Check sheet for the modelled part. Datum: model origin and axes. Units: mm. A direction names the side the tool comes from. Coordinates: 2 decimals unless noted, no trailing zeros. Write each loop counter-clockwise with the first axis right and the second up, starting at its lowest first coordinate (ties: lowest second). Pieces come first, ordered by that corner, then holes. Notation, with made-up numbers: M 62,51 L 66,51 A15 ccw 66,55 Z; hole C -18.5,-26 d11. An arc over 180 degrees is marked long. Answer as CSV lines item,"result". Start each with the question number.
1) Go/stop test with flat-tipped pins: pin 1 Ø10 at (x, z) = (-9.5, 1.5) entering from -Y; pin 2 Ø3 at (x, z) = (1.5, -3) entering from +Y; pin 3 Ø1.5 at (x, y) = (-16.5, -7.5) entering from -Z. Record where each tip stops, or that it passes through.
2) Access from +Z, -Z, +X, -X, +Y, -Y to the whole of each face (thin tool, end or side, straight path). Record for faces 1 (the flat face through (4, 4, -5.715)), 2 (the flat face through (-4, -4, -5.715)), 3 (the flat face through (4, -4, -5.715)), 4 (the cylindrical face through (1.18, -5.3, -9.41)), 5 (the flat face through (-5.429, 0, -3)).
3) Material ranges on L1, parallel to Y at x = 0, z = 23.95; L2, parallel to Y at x = 1, z = -4.5; L3, parallel to Z at x = 6, y = 1.5, recorded low to high. Write a range as [from, to].
4) Section check D-D (y = 2). Record the cut outline in (x, z) (3 decimals).
5) Section check B-B (y = 11.5). Record the cut outline in (x, z).
6) Draft check along Y on faces 6 (the cylindrical face through (-2.68, 20.4, 8.52)), 7 (the cylindrical face through (16.499, 5.196, 24.266)), 8 (the flat face through (4.59, -20.23, 17.272)), 9 (the flat face through (0, 0, 23.622)). Enter one of: +Y half, -Y half, draft (parallel to the pull), parting line (faces both ways), or undercut.
7) Section check A-A (x = -12). Record the cut outline in (y, z), and give its area (3 significant figures).
8) Section check C-C (z = -7.5). Record the cut outline in (x, y).
from build123d import *

# Parameters (mm, degrees)
SKETCH1_R           = 20.574
BOSS_EXTRUDE1_DEPTH = 24.892
SKETCH2_R           = 21.1074
BOSS_EXTRUDE2_DEPTH = 7.62
SKETCH3_R           = 17.2974
CUT_EXTRUDE1_DEPTH  = 1.27
SKETCH4_W           = 10.8585
SKETCH4_H           = 10.8585
BOSS_EXTRUDE3_DEPTH = 5.715
SKETCH5_R           = 5.42925
BOSS_EXTRUDE4_DEPTH = 7.493


with BuildPart() as part:
    # Sketch1 → Boss-Extrude1 (new body)
    with BuildSketch(Plane.XY):
        Circle(SKETCH1_R)
    extrude(amount=BOSS_EXTRUDE1_DEPTH)

    # Sketch2 → Boss-Extrude2 (add)
    with BuildSketch(Plane.XY.offset(24.892)):
        Circle(SKETCH2_R)
    extrude(amount=-BOSS_EXTRUDE2_DEPTH)

    # Sketch3 → Cut-Extrude1 (cut)
    with BuildSketch(Plane.XY.offset(24.892)):
        Circle(SKETCH3_R)
    extrude(amount=-CUT_EXTRUDE1_DEPTH, mode=Mode.SUBTRACT)

    # Sketch4 → Boss-Extrude3 (add)
    with BuildSketch(Plane(origin=(0, 0, 0), x_dir=(-1, 0, 0), z_dir=(0, 0, -1))):
        Rectangle(SKETCH4_W, SKETCH4_H)
    extrude(amount=BOSS_EXTRUDE3_DEPTH)

    # Sketch5 → Boss-Extrude4 (add)
    with BuildSketch(Plane(origin=(0, 0, -5.715), x_dir=(-1, 0, 0), z_dir=(0, 0, -1))):
        Circle(SKETCH5_R)
    extrude(amount=BOSS_EXTRUDE4_DEPTH)


solid = part.part
Results found:
1,pin 1,"stops at y = -20.08"
1,pin 2,"stops at y = 5.43"
1,pin 3,"stops at z = 0"
2,face 1,"-Z, +X, +Y"
2,face 2,"-Z, -X, -Y"
2,face 3,"-Z, +X, -Y"
2,face 4,"-Z"
2,face 5,"-Z, -X, +Y, -Y"
3,L1,"y = [-21.11, -17.3], [17.3, 21.11]"
3,L2,"y = [-5.43, 5.43]"
3,L3,"z = [0, 23.62]"
4,outline,"M -21.012,17.272 L -20.477,17.272 L -20.477,0 L -5.429,0 L -5.429,-5.715 L -5.047,-5.715 L -5.047,-13.208 L 5.047,-13.208 L 5.047,-5.715 L 5.429,-5.715 L 5.429,0 L 20.477,0 L 20.477,17.272 L 21.012,17.272 L 21.012,24.892 L 17.181,24.892 L 17.181,23.622 L -17.181,23.622 L -17.181,24.892 L -21.012,24.892 Z"
5,outline,"M -17.7,17.27 L -17.06,17.27 L -17.06,0 L 17.06,0 L 17.06,17.27 L 17.7,17.27 L 17.7,24.89 L 12.92,24.89 L 12.92,23.62 L -12.92,23.62 L -12.92,24.89 L -17.7,24.89 Z"
6,face 6,"parting line"
6,face 7,"undercut"
6,face 8,"draft"
6,face 9,"undercut"
7,outline,"M -17.36,17.27 L -16.71,17.27 L -16.71,0 L 16.71,0 L 16.71,17.27 L 17.36,17.27 L 17.36,24.89 L 12.46,24.89 L 12.46,23.62 L -12.46,23.62 L -12.46,24.89 L -17.36,24.89 Z"
7,area,"810 mm2"
8,outline,"C 0,0 d10.86"
